Could you check a few things on this drawing? It's one solid part, dimensions in mm from its lowest x, y, z. A direction names the side the tool comes from. Coordinates: 2 decimals unless noted, no trailing zeros. Order: outer loops, then holes, each group sorted by start corner. A loop starts at its lowest first (then second) coordinate and runs counter-clockwise, first axis right, second up. Notation, with made-up numbers: M 33.5,71 L 48.5,71 A20 cw 48.5,84 Z; hole C 58,12.25 d6. An arc over 180 degrees is marked long. Answer as CSV lines item,"result". Start each with the question number.
1. If we section it at C-C (x = 16): List the corners of the cut face in (y, z) for me (3 decimals).
2. I need wall thicknesses on line 1 along Z through (x, y) = (24, 3.9) (3 decimals); line 2 along Y through (x, z) = (12, 3.25); line 3 along X through (y, z) = (4.5, 5). Which ranges of each line are inside material? Lowest first, please. Write a range as from..to.
3. Will these pins go through, and if not, where does the flat tip stop? pin 1 (2.5 mm diameter, centred on y = 16, z = 3.175, fed in from -X); pin 2 (1.9 mm diameter, centred on y = 22.5, z = 2, fed in from +X); pin 3 (2.5 mm diameter, centred on y = 24, z = 3.175, fed in from +X).
4. On a 3-axis mill with a long thin cutter (end or side, diameter ignored), from which of +Z, -Z, +X, -X, +Y, -Y can I reach the whole of each face in a straight line? I mean the marked faces 1, 2 and 3. Say none if no direction works.
5. If we section it at A-A (x = 11): List the corners of the cut face in (y, z) for me.
6. If we mould it in two halves opening along Z, with no side actions, what happens to the marked faces 4, 5, 6 and 7? For each: released by +Z, released by -Z, zero draft, split by the parting line, or undercut.
7. If we section it at D-D (z = 4.75): Give the number of separate pieces and of enclosed holes in the cut face, plus the area to 3 significant figures.
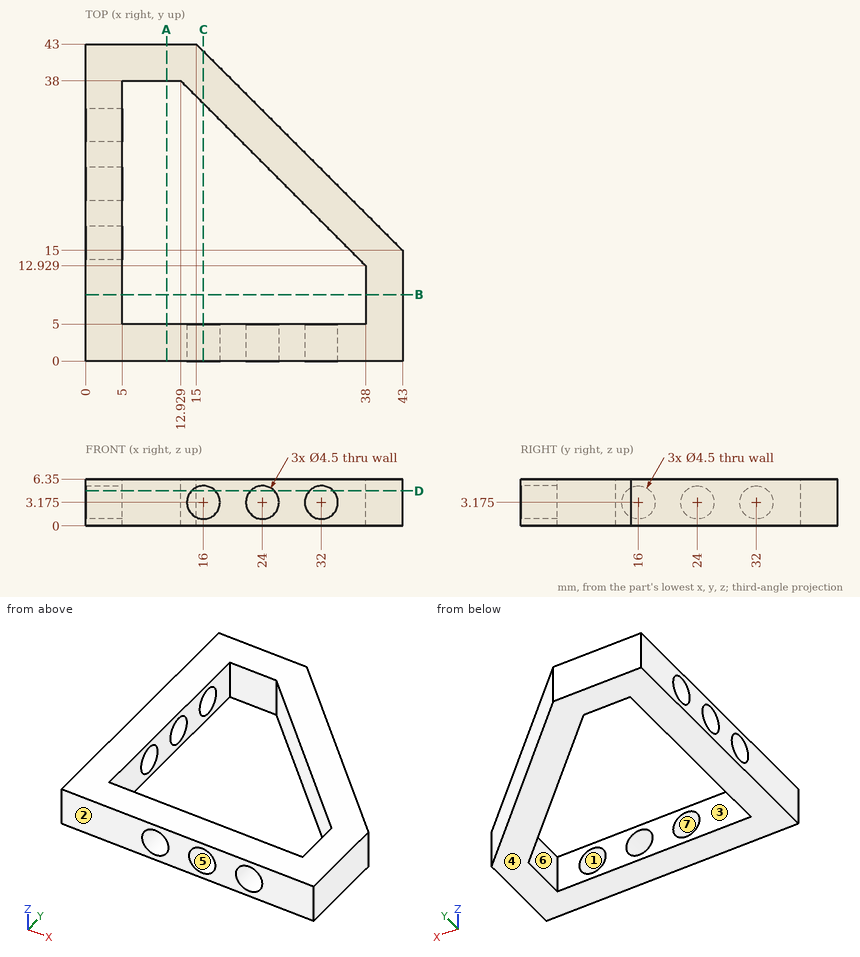
Solved:
1,outline,"M 0,0 L 5,0 L 5,0.925 L 0,0.925 Z; M 0,5.425 L 5,5.425 L 5,6.35 L 0,6.35 Z; M 34.929,0 L 42,0 L 42,6.35 L 34.929,6.35 Z"
2,line 1,"0..0.925, 5.425..6.35"
2,line 2,"0..5, 38..43"
2,line 3,"0..14.68, 17.32..22.68, 25.32..30.68, 33.32..43"
3,pin 1,"x = 33.68"
3,pin 2,"x = 36.45"
3,pin 3,"x = 35.25"
4,face 1,"-Y"
4,face 2,"+Z, -Z, +X, -X, -Y"
4,face 3,"+Z, -Z"
5,outline,"M 0,0 L 5,0 L 5,6.35 L 0,6.35 Z; M 38,0 L 43,0 L 43,6.35 L 38,6.35 Z"
6,face 4,"released by -Z"
6,face 5,"undercut"
6,face 6,"zero draft"
6,face 7,"undercut"
7,separate pieces,"6"
7,enclosed holes,"0"
7,area,"586 mm²"
